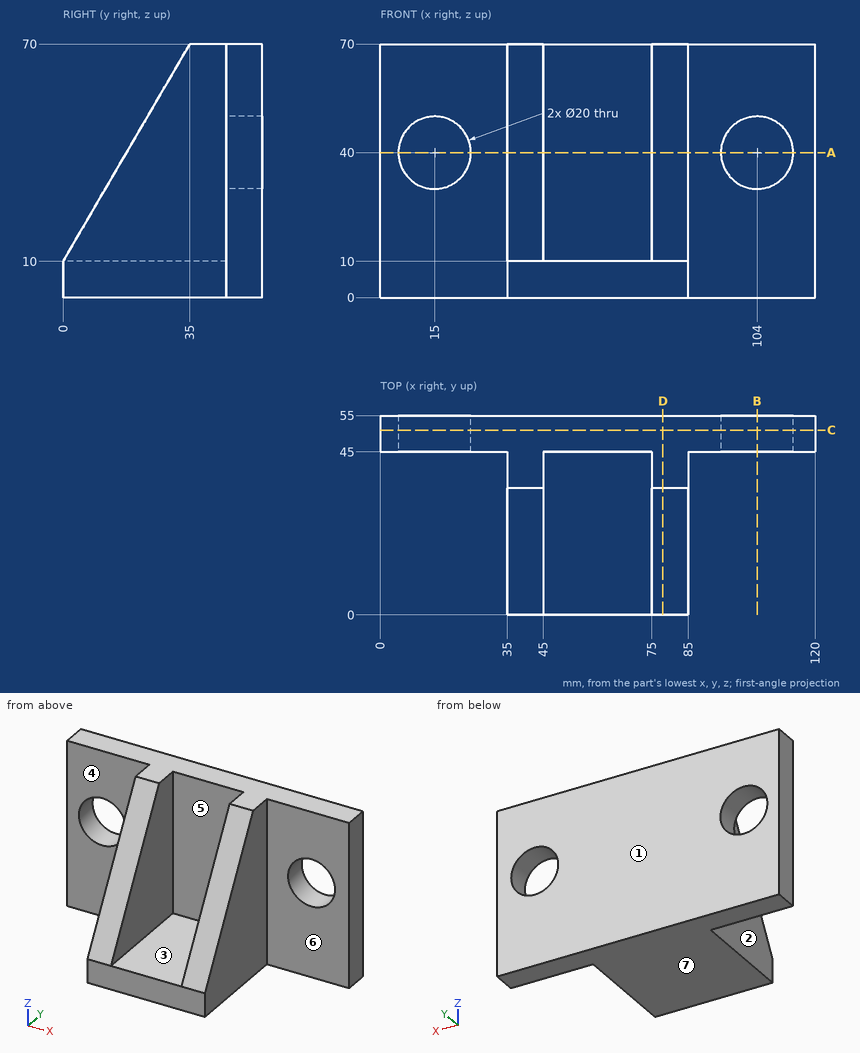
Geometry: see drawing. Coordinates: mm, zero at the bounding-box minimum. A direction names the side the tool comes from. Give positions to 0.01 mm unless a question says otherwise; leave off trailing zeros. Write each loop counter-clockwise with the first axis right and the second up, starting at its lowest first coordinate (ties: lowest second). Pieces come first, ordered by that corner, then holes. Notation, with made-up numbers: (65.5, 53.25) - (76.5, 53.25) arc R16 cw to (76.5, 83.25) - close; hole circle Ø2 at (82.5, 55). An arc over 180 degrees is marked (long way). Return JSON: item names as keys, results as strings. Group by question number.
1) Mould query, pull axis X, two halves, no side actions, for the marked faces 1, 2 and 3. Classes: released by +X, released by -X, zero draft, split by the parting line, or undercut.
2) Section C-C on y = 51. Return the cut outline in (x, z), plus the area to 3 significant figures.
3) Section D-D on x = 78. Return the cut outline in (y, z).
4) Line query: line 1 (X direction, y = 33.5, z = 57); line 2 (Z direction, x = 15, y = 48.5); line 3 (Y direction, x = 51.5, z = 54). Output: solid intervals per line, ascending.
5) Section B-B on x = 104. Return the cut outline in (y, z), plus the area to 3 significant figures.
6) Set-up query: the marked faces 4, 5, 6 and 7. Return all of +Z, -Z, +X, -X, +Y, -Y with unobstructed straight access to the full face (end or side cutting, diameter ignored); none if empty.
7) Section A-A on z = 40. Return the cut outline in (x, y), plus the area to 3 significant figures.
8) First-contact query: P1, Ø13.5, axis at y = 19, z = 49, coming from the -X side; P2, Ø23, axis at x = 15, z = 40, coming from the +Y side; P3, Ø15, axis at x = 67, z = 29, coming from the -Y side; P4, Ø13.5, axis at y = 28.5, z = 49.5, coming from the +X side. Flat tips, straight axial feed; report the tip coordinate or a pass-through.
Filled in:
{
 "1": {"face 1": "zero draft", "face 2": "released by -X", "face 3": "undercut"},
 "2": {"outline": "(0, 0) - (120, 0) - (120, 70) - (0, 70) - close; hole circle Ø20 at (15, 40); hole circle Ø20 at (104, 40)", "area": "7,770 mm^2"},
 "3": {"outline": "(0, 0) - (55, 0) - (55, 70) - (35, 70) - (0, 10) - close"},
 "4": {"line 1": "x = 35 to 45, 75 to 85", "line 2": "z = 0 to 30, 50 to 70", "line 3": "y = 45 to 55"},
 "5": {"outline": "(45, 0) - (55, 0) - (55, 30) - (45, 30) - close; (45, 50) - (55, 50) - (55, 70) - (45, 70) - close", "area": "500 mm^2"},
 "6": {"face 4": "+Z, -Z, -X, -Y", "face 5": "+Z, -Y", "face 6": "+Z, -Z, +X, -Y", "face 7": "-Z, +X, -X, +Y, -Y"},
 "7": {"outline": "(0, 45) - (5, 45) - (5, 55) - (0, 55) - close; (25, 45) - (35, 45) - (35, 17.5) - (45, 17.5) - (45, 45) - (75, 45) - (75, 17.5) - (85, 17.5) - (85, 45) - (94, 45) - (94, 55) - (25, 55) - close; (114, 45) - (120, 45) - (120, 55) - (114, 55) - close", "area": "1,350 mm^2"},
 "8": {"P1": "stops at x = 35", "P2": "stops at y = 55", "P3": "stops at y = 45", "P4": "stops at x = 85"}
}
